The model under review builds one solid part; all positions refer to its coordinate system, in mm. Round coordinates to 2 decimals unless told otherwise and drop trailing zeros. Order: outer loops, then holes, each group sorted by start corner. A loop starts at its lowest first (then second) coordinate and runs counter-clockwise, first axis right, second up. Notation, with made-up numbers: M 60,5 L 85,5 A28 cw 85,25 Z; hole C 35,88 d5. An arc over 180 degrees is marked long. Use a Markdown table: item, result. Add a question column.
1. To check wall thickness, follow probe 1 along Z at (x, y) = (2.6, 0.8); probe 2 along Y at (x, z) = (0.3, 96); probe 3 along X at (y, z) = (2.7, 76). State the ranges of each line that lie inside material, in increasing order.
2. Consider section A-A on y = -0.9. State the section outline as (x, z) points, then the cut area to 3 significant figures.
3. Consider section C-C on x = 0.5. State the section outline as (y, z) points.
4. Consider section B-B on z = 15. State the section outline as (x, y) points.
5. Insertion check: P1, Ø1.5, axis at x = 0.5, y = -2.5, coming from the -Z side; P2, Ø0.5, axis at y = 0.5, z = -0.5, coming from the +X side; P3, Ø1.1, axis at y = 0.5, z = -0.5, coming from the -X side; P4, Ø0.7, axis at x = -2.5, y = -0.5, coming from the +Z side. Each pin has a flat end and moves straight along its axis. Give the tip position at first contact, or say it passes through.
from build123d import *

# Parameters (mm, degrees)
MAIN_BAR_CROSS_SECTION_R = 3
BOSS_EXTRUDE1_DEPTH      = 102
SKETCH2_W                = 4.242640688
SKETCH2_H                = 4.242640688
BOSS_EXTRUDE2_DEPTH      = 1
SKETCH3_W                = 4.24
SKETCH3_H                = 4.245279732
BOSS_EXTRUDE3_DEPTH      = 1


with BuildPart() as part:
    # Main bar cross section → Boss-Extrude1 (new body)
    with BuildSketch(Plane.XY):
        Circle(MAIN_BAR_CROSS_SECTION_R)
    extrude(amount=BOSS_EXTRUDE1_DEPTH)

    # Sketch2 → Boss-Extrude2 (add)
    with BuildSketch(Plane(origin=(0, 0, 0), x_dir=(-1, 0, 0), z_dir=(0, 0, -1))):
        Rectangle(SKETCH2_W, SKETCH2_H)
    extrude(amount=BOSS_EXTRUDE2_DEPTH)

    # Sketch3 → Boss-Extrude3 (add)
    with BuildSketch(Plane.XY.offset(102)):
        Rectangle(SKETCH3_W, SKETCH3_H)
    extrude(amount=BOSS_EXTRUDE3_DEPTH)


solid = part.part
Answer block:
| question | item | result |
|---|---|---|
| 1 | probe 1 | 0 to 102 |
| 1 | probe 2 | -2.98 to 2.98 |
| 1 | probe 3 | -1.31 to 1.31 |
| 2 | outline | M -2.86,0 L -2.12,0 L -2.12,-1 L 2.12,-1 L 2.12,0 L 2.86,0 L 2.86,102 L 2.12,102 L 2.12,103 L -2.12,103 L -2.12,102 L -2.86,102 Z |
| 2 | area | 592 mm^2 |
| 3 | outline | M -2.96,0 L -2.12,0 L -2.12,-1 L 2.12,-1 L 2.12,0 L 2.96,0 L 2.96,102 L 2.12,102 L 2.12,103 L -2.12,103 L -2.12,102 L -2.96,102 Z |
| 4 | outline | C 0,0 d6 |
| 5 | P1 | z = -1 |
| 5 | P2 | x = 2.12 |
| 5 | P3 | x = -2.99 |
| 5 | P4 | z = 102 |
